Verification items for the finished model (mm, model axes). A direction names the side the tool comes from. Give positions to 0.01 mm unless a question says otherwise; leave off trailing zeros. Loops run counter-clockwise (first coordinate to the right, second up) from the corner with the lowest first, then second, coordinate; pieces in that order, holes last. Notation, with made-up numbers: (-18.75, 2) - (8.25, 2) arc R31 ccw to (8.25, 32) - close; hole circle Ø7 at (76, -21). An arc over 180 degrees is marked (long way). One line per item, written item: value. Start each with the question number.
1. Sectioned sample at D-D (y = 6). Record the cut outline in (x, z), plus the area to 3 significant figures.
2. Sectioned sample at B-B (z = 11.25). Record the cut outline in (x, y), plus the area to 3 significant figures.
3. Gauge pin test, flat ends, axial feed: pin 1 (1.5 mm diameter, centred on x = 9.5, y = 5, fed in from +Z); pin 2 (1 mm diameter, centred on x = 4.5, z = 10.5, fed in from -Y); pin 3 (2 mm diameter, centred on x = -7.5, z = 5, fed in from -Y); pin 4 (4 mm diameter, centred on y = 3, z = 4, fed in from +X). Record the tip position at first contact, or that the pin passes through.
4. Scan lines: L1, parallel to X at y = -5, z = 11.2; L2, parallel to Y at x = -10, z = 11.05; L3, parallel to X at y = -5.5, z = 11. Record each from-to range of solid material in increasing order. Write a range as [from, to].
5. Sectioned sample at C-C (y = 0). Record the cut outline in (x, z), plus the area to 4 significant figures.
6. Sectioned sample at A-A (z = 6). Record the cut outline in (x, y), plus the area to 3 significant figures.
7. Access from +Z, -Z, +X, -X, +Y, -Y to the whole of each face (thin tool, end or side, straight path). Record for faces 1 (the flat face through (-10.41, -7.6, 3.47)), 2 (the flat face through (-10, -5, 10.1)), 3 (the flat face through (-10.41, 7.6, 3.47)), 4 (the flat face through (10.4, -6, 1.6)), 5 (the flat face through (-11.79, 5.22, 3.47)).
8. Mould release check, pull along Z, two halves, no side actions. Record for faces 6 (the flat face through (11.79, -5.22, 3.47)), 7 (the flat face through (10.618, 6.108, 4.188)), 8 (the flat face through (10.4, 6, 1.6)), 9 (the flat face through (-10.8, 6.21, 0.79)): pulls with the +Z half, pulls with the -Z half, needs draft (parallel to the pull), parting line crosses it, or undercut.
from build123d import *

# Parameters (mm, degrees)
SKETCH002_R                = 13
PAD001_DEPTH               = 5.25
SKETCH012_R                = 1.5
POCKET003_DEPTH            = 2
SKETCH012_MIRRORED_2_R     = 1.5
POCKET003_MIRRORED_2_DEPTH = 2
PAD007_DEPTH               = 1.375
PAD007_MIRRORED002_2_DEPTH = 1.375


with BuildPart() as part:
    # Sketch002 → Pad001 (new body)
    with BuildSketch(Plane(origin=(0, 0, 6.85), x_dir=(0, 1, 0), z_dir=(0, 0, 1))):
        Circle(SKETCH002_R)
    extrude(amount=PAD001_DEPTH)

    # Sketch012 (on Face3 of Pad001) → Pocket003 (cut)
    with BuildSketch(Plane(origin=(-10, 5, 12.1), x_dir=(1, 0, 0), z_dir=(0, 0, 1))):
        Circle(SKETCH012_R)
    pocket003 = extrude(amount=-POCKET003_DEPTH, mode=Mode.SUBTRACT)

    # Sketch012 Mirrored 2 → Pocket003 Mirrored 2 (cut)
    with BuildSketch(Plane(origin=(10, 5, 12.1), x_dir=(-1, 0, 0), z_dir=(0, 0, -1))):
        Circle(SKETCH012_MIRRORED_2_R)
    pocket003_mirrored_2 = extrude(amount=POCKET003_MIRRORED_2_DEPTH, mode=Mode.SUBTRACT)

    # Mirrored001: Pocket003, Pocket003 Mirrored 2 across XZ
    add(pocket003.mirror(Plane.XZ), mode=Mode.SUBTRACT)
    add(pocket003_mirrored_2.mirror(Plane.XZ), mode=Mode.SUBTRACT)

    # Sketch013 → Pad007 (join, symmetric)
    with BuildSketch(Plane(origin=(0, 0, 0), x_dir=(0.866025, 0.5, 0), z_dir=(0.5, -0.866025, 0))):
        Polygon((13.25, 6.85), (13.25, 0), (11.65, 1.6), (12.25, 1.6), (12.25, 6.85), align=None)
    pad007 = extrude(amount=PAD007_DEPTH, both=True)

    # Sketch013 Mirrored002 2 → Pad007 Mirrored002 2 (add, symmetric)
    with BuildSketch(Plane(origin=(0, 0, 0), x_dir=(0.866025, -0.5, 0), z_dir=(-0.5, -0.866025, 0))):
        Polygon((13.25, 6.85), (13.25, 0), (11.65, 1.6), (12.25, 1.6), (12.25, 6.85), align=None)
    pad007_mirrored002_2 = extrude(amount=-PAD007_MIRRORED002_2_DEPTH, both=True)

    # Mirrored003: Pad007, Pad007 Mirrored002 2 across YZ
    add(pad007.mirror(Plane.YZ))
    add(pad007_mirrored002_2.mirror(Plane.YZ))


solid = part.part
Results are:
1. outline: (-11.84, 0) - (-9.99, 1.6) - (-10.68, 1.6) - (-10.68, 6.85) - (10.68, 6.85) - (10.68, 1.6) - (9.99, 1.6) - (11.84, 0) - (11.84, 6.85) - (11.53, 6.85) - (11.53, 12.1) - (11.12, 12.1) - (11.12, 10.1) - (8.88, 10.1) - (8.88, 12.1) - (-8.88, 12.1) - (-8.88, 10.1) - (-11.12, 10.1) - (-11.12, 12.1) - (-11.53, 12.1) - (-11.53, 6.85) - (-11.84, 6.85) - close
1. area: 127 mm^2
2. outline: circle Ø26 at (0, 0); hole circle Ø3 at (-10, -5); hole circle Ø3 at (-10, 5); hole circle Ø3 at (10, -5); hole circle Ø3 at (10, 5)
2. area: 503 mm^2
3. pin 1: stops at z = 10.1
3. pin 2: stops at y = -12.37
3. pin 3: passes through
3. pin 4: stops at x = 11.41
4. L1: x = [-12, -11.5], [-8.5, 8.5], [11.5, 12]
4. L2: y = [-8.31, -6.5], [-3.5, 3.5], [6.5, 8.31]
4. L3: x = [-11.78, -11.41], [-8.59, 8.59], [11.41, 11.78]
5. outline: (-13, 6.85) - (13, 6.85) - (13, 12.1) - (-13, 12.1) - close
5. area: 136.5 mm^2
6. outline: (-12.16, -5.43) - (-10.79, -7.82) - (-9.92, -7.32) - (-11.3, -4.93) - close; (-12.16, 5.43) - (-11.3, 4.93) - (-9.92, 7.32) - (-10.79, 7.82) - close; (9.92, -7.32) - (10.79, -7.82) - (12.16, -5.43) - (11.3, -4.93) - close; (9.92, 7.32) - (11.3, 4.93) - (12.16, 5.43) - (10.79, 7.82) - close
6. area: 11.0 mm^2
7. face 1: -Z, -Y
7. face 2: +Z
7. face 3: -Z, +Y
7. face 4: none
7. face 5: -Z, -X
8. face 6: needs draft
8. face 7: undercut
8. face 8: undercut
8. face 9: pulls with the -Z half
